Work out the finished part from the listing and answer in its coordinate system (mm). Face numbers are marked on the shaded views. A direction names the side the tool comes from. Coordinates: 2 decimals unless noted, no trailing zeros. Order: outer loops, then holes, each group sorted by start corner. A loop starts at its lowest first (then second) coordinate and runs counter-clockwise, first axis right, second up. Notation, with made-up numbers: (20, 10.25) - (77, 10.25) arc R8 cw to (77, 17.25) - close; hole circle Ø7 at (87, -6). An arc over 180 degrees is marked (long way). Answer as a JSON object with one key per item and string values. Group by question number.
1) The mould has two halves that part along Y. Classify the marked faces 1, 2 and 3: released by +Y, released by -Y, zero draft, split by the parting line, or undercut.
2) Section A-A (y = 0) is taken. Give the vertices of the cut face in (x, z), plus the area to 3 significant figures.
3) Find the intervals of material crossed by line 1 along X through (y, z) = (0.5, 6.25); line 2 along Y through (x, z) = (0, 6.3); line 3 along X through (y, z) = (-18.5, 3.75), in increasing order.
4) Section B-B (x = 22.5) is taken. Give the vertices of the cut face in (y, z), plus the area to 3 significant figures.
5) Section D-D (x = -18.42) is taken. Give the vertices of the cut face in (y, z).
6) A tool of negligible diameter and unlimited length cuts with its end or side. For the marked faces 4, 5, 6, 7 and 8, from which of +Z, -Z, +X, -X, +Y, -Y can it reach the whole face along a straight path? Write none if from no direction.
7) Each of these flat-tipped pins is pushed along its axis until it touches: P1, Ø1.6, axis at x = 26.91, z = 1.7, coming from the -Y side; P2, Ø4, axis at x = -11, y = 21, coming from the -Z side; P3, Ø1.5, axis at x = 26.5, z = 2.5, coming from the +Y side; P4, Ø10, axis at x = -3, y = 2.5, coming from the -Z side. Where does it stop, or does it pass through?
8) Section C-C (y = -10.5) is taken. Give the vertices of the cut face in (x, z), plus the area to 3 significant figures.
from build123d import *

# Parameters (mm, degrees)
PAD_DEPTH       = 6.5
POCKET_DEPTH    = 6
SKETCH002_R     = 13.5
POCKET001_DEPTH = 1
SKETCH003_W     = 5.4
SKETCH003_H     = 6.5
PAD001_DEPTH    = 3
POCKET002_DEPTH = 10
SKETCH008_R     = 0.6
POCKET003_DEPTH = 2
SKETCH009_R     = 0.6
POCKET004_DEPTH = 2
FILLET_R        = 2.9
FILLET001_R     = 2.9
FILLET002_R     = 5
FILLET003_R     = 5
FILLET004_R     = 5
FILLET005_R     = 5
SKETCH010_W     = 3.95
SKETCH010_H     = 6.5
PAD002_DEPTH    = 3.5
POCKET005_DEPTH = 10
SKETCH012_R     = 0.6
POCKET006_DEPTH = 2
SKETCH013_R     = 0.6
POCKET007_DEPTH = 2
FILLET006_R     = 3.4
FILLET007_R     = 3.4
SKETCH014_R     = 20.45
SKETCH014_R_2   = 19.5
POCKET008_DEPTH = 0.3
SKETCH015_R     = 0.9
PAD003_DEPTH    = 6
FILLET008_R     = 1
POCKET009_DEPTH = 4
POCKET010_DEPTH = 4


with BuildPart() as part:
    # Sketch → Pad (new body)
    with BuildSketch(Plane.XY):
        with BuildLine():
            Line((-22.5019915649, 16), (-22.5019915649, -16))
            Line((-22.5019915649, -16), (-16.2858834578, -17.9))
            ThreePointArc((-16.2858834578, -17.9), (0.2206895736, -24.1989937004), (16.6096357576, -17.6))
            Line((16.6096357576, -17.6), (25.6083856708, -17.45))
            Line((25.6083856708, 17.45), (25.6083856708, -17.45))
            Line((16.6096357576, 17.6), (25.6083856708, 17.45))
            ThreePointArc((16.6096357576, 17.6), (0.2206895736, 24.1989937004), (-16.2858834578, 17.9))
            Line((-22.5019915649, 16), (-16.2858834578, 17.9))
        make_face()
    extrude(amount=PAD_DEPTH)

    # Sketch001 → Pocket (cut)
    with BuildSketch(Plane.XY):
        with BuildLine():
            Line((-15.2429491897, 16.55), (-20.5746937447, 15.2))
            Line((-20.5746937447, 15.2), (-20.5746937447, -15.2))
            Line((-20.5746937447, -15.2), (-15.2429491897, -16.55))
            ThreePointArc((-15.2429491897, -16.55), (0, -22.5), (15.2429491897, -16.55))
            Line((15.2429491897, -16.55), (23.5278752606, -16.05))
            Line((23.5278752606, 16.05), (23.5278752606, -16.05))
            Line((15.2429491897, 16.55), (23.5278752606, 16.05))
            ThreePointArc((15.2429491897, 16.55), (0, 22.5), (-15.2429491897, 16.55))
        make_face()
    extrude(amount=POCKET_DEPTH, mode=Mode.SUBTRACT)

    # Sketch002 (on Face19 of Pocket) → Pocket001 (cut)
    with BuildSketch(Plane(origin=(0, 0, 6), x_dir=(1, 0, 0), z_dir=(0, 0, -1))):
        Circle(SKETCH002_R)
    extrude(amount=-POCKET001_DEPTH, mode=Mode.SUBTRACT)

    # Sketch003 (on Face6 of Pocket001) → Pad001 (join)
    with BuildSketch(Plane.YZ.offset(25.6083856708)):
        with Locations((-14.75, 3.25)):
            Rectangle(SKETCH003_W, SKETCH003_H)
        with Locations((14.75, 3.25)):
            Rectangle(SKETCH003_W, SKETCH003_H)
    extrude(amount=PAD001_DEPTH)

    # Sketch006 → Pocket002 (cut)
    with BuildSketch(Plane.XY.offset(6.5)):
        with BuildLine():
            ThreePointArc((25.6083856708, 17.45), (27.0135397777, 16.4426436477), (28.6083856708, 15.775042373))
            Line((28.6083856708, 17.45), (28.6083856708, 15.775042373))
            Line((28.6083856708, 17.45), (25.6083856708, 17.45))
        make_face()
        with BuildLine():
            ThreePointArc((28.6083856708, -15.775042373), (27.0135397777, -16.4426436477), (25.6083856708, -17.45))
            Line((28.6083856708, -17.45), (25.6083856708, -17.45))
            Line((28.6083856708, -15.775042373), (28.6083856708, -17.45))
        make_face()
    extrude(amount=-POCKET002_DEPTH, mode=Mode.SUBTRACT)

    # Sketch008 (on Face27 of Pocket002) → Pocket003 (cut)
    with BuildSketch(Plane(origin=(0, -12.05, 0), x_dir=(-1, 0, 0), z_dir=(0, 1, 0))):
        with Locations((-26.9083856708, 1.7)):
            Circle(SKETCH008_R)
    extrude(amount=-POCKET003_DEPTH, mode=Mode.SUBTRACT)

    # Sketch009 (on Face26 of Pocket003) → Pocket004 (cut)
    with BuildSketch(Plane.XZ.offset(-12.05)):
        with Locations((26.9083856708, 1.7)):
            Circle(SKETCH009_R)
    extrude(amount=-POCKET004_DEPTH, mode=Mode.SUBTRACT)

    # Fillet
    fillet_edges = [part.edges().sort_by_distance(p)[0] for p in [
        (28.608386, -13.912521, 6.5),
    ]]
    fillet(fillet_edges, radius=FILLET_R)

    # Fillet001
    fillet001_edges = [part.edges().sort_by_distance(p)[0] for p in [
        (28.608386, 13.912521, 6.5),
    ]]
    fillet(fillet001_edges, radius=FILLET001_R)

    # Fillet002
    fillet002_edges = [part.edges().sort_by_distance(p)[0] for p in [
        (16.609636, -17.6, 3.25),
    ]]
    fillet(fillet002_edges, radius=FILLET002_R)

    # Fillet003
    fillet003_edges = [part.edges().sort_by_distance(p)[0] for p in [
        (16.609636, 17.6, 3.25),
    ]]
    fillet(fillet003_edges, radius=FILLET003_R)

    # Fillet004
    fillet004_edges = [part.edges().sort_by_distance(p)[0] for p in [
        (-16.285883, -17.9, 3.25),
    ]]
    fillet(fillet004_edges, radius=FILLET004_R)

    # Fillet005
    fillet005_edges = [part.edges().sort_by_distance(p)[0] for p in [
        (-16.285883, 17.9, 3.25),
    ]]
    fillet(fillet005_edges, radius=FILLET005_R)

    # Sketch010 (on Face4 of Fillet005) → Pad002 (join)
    with BuildSketch(Plane(origin=(-22.5019915649, 0, 0), x_dir=(0, -1, 0), z_dir=(-1, 0, 0))):
        with Locations((-14.025, 3.25)):
            Rectangle(SKETCH010_W, SKETCH010_H)
        with Locations((14.025, 3.25)):
            Rectangle(SKETCH010_W, SKETCH010_H)
    extrude(amount=PAD002_DEPTH)

    # Sketch011 (on Face6 of Pad002) → Pocket005 (cut)
    with BuildSketch(Plane.XY.offset(6.5)):
        with BuildLine():
            ThreePointArc((-26.0019915649, 14.6), (-24.1926075875, 15.1515400564), (-22.5019915649, 16))
            Line((-22.5019915649, 16), (-26.0019915649, 16))
            Line((-26.0019915649, 16), (-26.0019915649, 14.6))
        make_face()
        with BuildLine():
            ThreePointArc((-22.5019915649, -16), (-24.1926075875, -15.1515400564), (-26.0019915649, -14.6))
            Line((-26.0019915649, -14.6), (-26.0019915649, -16))
            Line((-26.0019915649, -16), (-22.5019915649, -16))
        make_face()
    extrude(amount=-POCKET005_DEPTH, mode=Mode.SUBTRACT)

    # Sketch012 (on Face23 of Pocket005) → Pocket006 (cut)
    with BuildSketch(Plane(origin=(0, -12.05, 0), x_dir=(-1, 0, 0), z_dir=(0, 1, 0))):
        with Locations((24.3019915649, 1.7)):
            Circle(SKETCH012_R)
    extrude(amount=-POCKET006_DEPTH, mode=Mode.SUBTRACT)

    # Sketch013 (on Face21 of Pocket006) → Pocket007 (cut)
    with BuildSketch(Plane.XZ.offset(-12.05)):
        with Locations((-24.3019915649, 1.7)):
            Circle(SKETCH013_R)
    extrude(amount=-POCKET007_DEPTH, mode=Mode.SUBTRACT)

    # Fillet006
    fillet006_edges = [part.edges().sort_by_distance(p)[0] for p in [
        (-26.001992, 13.325, 6.5),
    ]]
    fillet(fillet006_edges, radius=FILLET006_R)

    # Fillet007
    fillet007_edges = [part.edges().sort_by_distance(p)[0] for p in [
        (-26.001992, -13.325, 6.5),
    ]]
    fillet(fillet007_edges, radius=FILLET007_R)

    # Sketch014 (on Face4 of Fillet007) → Pocket008 (cut)
    with BuildSketch(Plane.XY.offset(6.5)):
        Circle(SKETCH014_R)
        Circle(SKETCH014_R_2, mode=Mode.SUBTRACT)
    extrude(amount=-POCKET008_DEPTH, mode=Mode.SUBTRACT)

    # Sketch015 (on Face55 of Pocket008) → Pad003 (join)
    with BuildSketch(Plane(origin=(0, 0, 6), x_dir=(1, 0, 0), z_dir=(0, 0, -1))):
        with Locations((-18.42, 13.32)):
            Circle(SKETCH015_R)
        with Locations((-18.42, -13.32)):
            Circle(SKETCH015_R)
        with Locations((7.27, 18.56)):
            Circle(SKETCH015_R)
        with Locations((5.37, -19.79)):
            Circle(SKETCH015_R)
    extrude(amount=PAD003_DEPTH)

    # Fillet008
    fillet008_edges = [part.edges().sort_by_distance(p)[0] for p in [
        (-19.32, -13.32, 6),
        (6.37, -18.56, 6),
        (-19.32, 13.32, 6),
        (4.47, 19.79, 6),
    ]]
    fillet(fillet008_edges, radius=FILLET008_R)

    # Sketch016 (on Face16 of Fillet008) → Pocket009 (cut)
    with BuildSketch(Plane(origin=(0, 0, 0), x_dir=(1, 0, 0), z_dir=(0, 0, -1))):
        with BuildLine():
            Line((-5, 23.6778377391), (-5, 21.9374109685))
            ThreePointArc((5, 21.9374109685), (0, 22.5), (-5, 21.9374109685))
            Line((5, 23.6778377391), (5, 21.9374109685))
            ThreePointArc((5, 23.6778377391), (0, 24.2), (-5, 23.6778377391))
        make_face()
    extrude(amount=-POCKET009_DEPTH, mode=Mode.SUBTRACT)

    # Sketch017 (on Face16 of Pocket009) → Pocket010 (cut)
    with BuildSketch(Plane(origin=(0, 0, 0), x_dir=(1, 0, 0), z_dir=(0, 0, -1))):
        with BuildLine():
            Line((-3.499984119, -22.2261132717), (-3.5, -23.9455632634))
            ThreePointArc((-3.5, -23.9455632634), (0, -24.2000019575), (3.5, -23.9455632634))
            Line((3.5000158811, -22.2261082701), (3.5, -23.9455632634))
            ThreePointArc((-3.499984119, -22.2261132717), (1.60767e-05, -22.5), (3.5000158811, -22.2261082701))
        make_face()
        with BuildLine():
            ThreePointArc((-13.9498796389, -17.6536358312), (-11.25, -19.4855715851), (-8.3135572795, -20.9077680626))
            Line((-8.3135572795, -20.9077680626), (-8.9416927184, -22.487466094))
            ThreePointArc((-15.0038705449, -18.987466094), (-12.1, -20.9578147716), (-8.9416927184, -22.487466094))
            Line((-13.9498796389, -17.6536358312), (-15.0038705449, -18.987466094))
        make_face()
        with BuildLine():
            ThreePointArc((8.3135572795, -20.9077680626), (11.25, -19.4855715851), (13.9498796389, -17.6536358312))
            Line((13.9498796389, -17.6536358312), (15.0038705449, -18.987466094))
            ThreePointArc((8.9416927184, -22.487466094), (12.1, -20.9578147716), (15.0038705449, -18.987466094))
            Line((8.3135572795, -20.9077680626), (8.9416927184, -22.487466094))
        make_face()
    extrude(amount=-POCKET010_DEPTH, mode=Mode.SUBTRACT)


solid = part.part
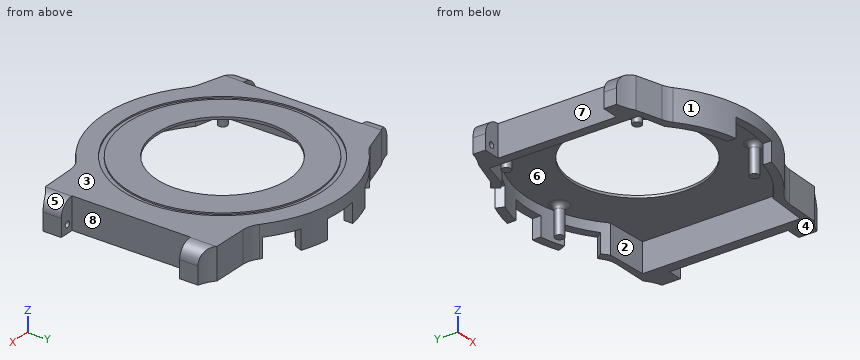
Report:
{
 "1": {"face 1": "released by -Y", "face 2": "undercut", "face 3": "zero draft"},
 "2": {"outline": "(-22.5, 0) - (-20.57, 0) - (-20.57, 6) - (-13.5, 6) - (-13.5, 6.5) - (-19.5, 6.5) - (-19.5, 6.2) - (-20.45, 6.2) - (-20.45, 6.5) - (-22.5, 6.5) - close; (13.5, 6) - (23.53, 6) - (23.53, 0) - (25.61, 0) - (25.61, 6.5) - (20.45, 6.5) - (20.45, 6.2) - (19.5, 6.2) - (19.5, 6.5) - (13.5, 6.5) - close", "area": "34.0 mm²"},
 "3": {"line 1": "x = -22.5 to -20.44, -19.49 to -13.49, 13.49 to 19.49, 20.44 to 25.61", "line 2": "y = -24.2 to -20.45, -19.5 to -13.5, 13.5 to 19.5, 20.45 to 24.2", "line 3": "x = -15.6 to -12.81, 6.37 to 8.17, 12.81 to 15.62"},
 "4": {"outline": "(-17.5, 0) - (-16.11, 0) - (-16.11, 6) - (16.11, 6) - (16.11, 0) - (17.5, 0) - (17.5, 6.5) - (-17.5, 6.5) - close", "area": "34.2 mm²"},
 "5": {"outline": "(-17.25, 0) - (-15.75, 0) - (-15.75, 6) - (-15.22, 6) arc R1 cw to (-14.22, 5) - (-14.22, 0) - (-12.42, 0) - (-12.42, 5) arc R1 cw to (-11.42, 6) - (11.42, 6) arc R1 cw to (12.42, 5) - (12.42, 0) - (14.22, 0) - (14.22, 5) arc R1 cw to (15.22, 6) - (15.75, 6) - (15.75, 0) - (17.25, 0) - (17.25, 6.5) - (8.88, 6.5) - (8.88, 6.2) - (6.4, 6.2) - (6.4, 6.5) - (-6.4, 6.5) - (-6.4, 6.2) - (-8.88, 6.2) - (-8.88, 6.5) - (-17.25, 6.5) - close"},
 "6": {"face 4": "-Z, +X, -X, +Y, -Y", "face 5": "+Z, +X, +Y, -Y", "face 6": "-Z", "face 7": "+Z, -Z, -X", "face 8": "+Z, -Z, +X"},
 "7": {"P1": "stops at y = -17.03", "P2": "stops at z = 4", "P3": "stops at y = 17.33", "P4": "passes through"},
 "8": {"outline": "(-22.5, 0) - (-20.57, 0) - (-20.57, 6) - (-8.49, 6) - (-8.49, 6.5) - (-16.43, 6.5) - (-16.43, 6.2) - (-17.55, 6.2) - (-17.55, 6.5) - (-22.5, 6.5) - close; (8.49, 6) - (23.53, 6) - (23.53, 0) - (25.61, 0) - (25.61, 6.5) - (17.55, 6.5) - (17.55, 6.2) - (16.43, 6.2) - (16.43, 6.5) - (8.49, 6.5) - close", "area": "38.9 mm²"}
}
